```python
from build123d import *

# Parameters (mm, degrees)
SKETCH_1_R      = 1.05
SKETCH_1_W      = 7
SKETCH_1_H      = 5
SKETCH_1_W_2    = 5
SKETCH_1_H_2    = 11
SKETCH_1_W_3    = 21
SKETCH_1_H_3    = 2
SKETCH_1_R_2    = 8.5
EXTRUDE_1_DEPTH = 1.6


with BuildPart() as part:
    # 草图1 → 凸台-拉伸1 (new body)
    with BuildSketch(Plane(origin=(0, 0, 0), x_dir=(1, 0, 0), z_dir=(0, 1, 0))):
        Polygon((99, 0), (0, 0), (0, -143), (99, -143), (99, -93), (93, -93), (93, -80.5), (99, -80.5), align=None)
        with Locations(Location((21.8, -94.8, 0), (0, 0, 270))):
            Circle(SKETCH_1_R, mode=Mode.SUBTRACT)
        with Locations((73, -90.5)):
            Rectangle(SKETCH_1_W, SKETCH_1_H, mode=Mode.SUBTRACT)
        with Locations(Location((71.4, -77.5, 0), (0, 0, 270))):
            Circle(SKETCH_1_R, mode=Mode.SUBTRACT)
        with Locations(Location((94.8, -94.8, 0), (0, 0, 270))):
            Circle(SKETCH_1_R, mode=Mode.SUBTRACT)
        with Locations(Location((8.7, -65.7, 0), (0, 0, 270))):
            Circle(SKETCH_1_R, mode=Mode.SUBTRACT)
        with Locations((38, -39)):
            Rectangle(SKETCH_1_W_2, SKETCH_1_H_2, mode=Mode.SUBTRACT)
        with Locations(Location((21.8, -26.8, 0), (0, 0, 270))):
            Circle(SKETCH_1_R, mode=Mode.SUBTRACT)
        with Locations(Location((7, -7, 0), (0, 0, 270))):
            Circle(SKETCH_1_R, mode=Mode.SUBTRACT)
        with Locations(Location((20, -12, 0), (0, 0, 270))):
            Circle(SKETCH_1_R, mode=Mode.SUBTRACT)
        with Locations((24.5, -3)):
            Rectangle(SKETCH_1_W_3, SKETCH_1_H_3, mode=Mode.SUBTRACT)
        with Locations(Location((50, -36.3, 0), (0, 0, 270))):
            Circle(SKETCH_1_R_2, mode=Mode.SUBTRACT)
        with Locations(Location((96.3, -55.2, 0), (0, 0, 270))):
            Circle(SKETCH_1_R, mode=Mode.SUBTRACT)
        with Locations(Location((94.8, -26.8, 0), (0, 0, 270))):
            Circle(SKETCH_1_R, mode=Mode.SUBTRACT)
        with Locations(Location((81.9, -4.6, 0), (0, 0, 270))):
            Circle(SKETCH_1_R, mode=Mode.SUBTRACT)
        with Locations(Location((87, -7, 0), (0, 0, 270))):
            Circle(SKETCH_1_R, mode=Mode.SUBTRACT)
        with Locations(Location((66, -106, 0), (0, 0, 270))):
            Circle(SKETCH_1_R, mode=Mode.SUBTRACT)
        with Locations(Location((7, -136, 0), (0, 0, 270))):
            Circle(SKETCH_1_R, mode=Mode.SUBTRACT)
        with Locations(Location((33, -132, 0), (0, 0, 270))):
            Circle(SKETCH_1_R, mode=Mode.SUBTRACT)
        with Locations(Location((33, -106, 0), (0, 0, 270))):
            Circle(SKETCH_1_R, mode=Mode.SUBTRACT)
        with Locations(Location((66, -132, 0), (0, 0, 270))):
            Circle(SKETCH_1_R, mode=Mode.SUBTRACT)
        with Locations(Location((87, -136, 0), (0, 0, 270))):
            Circle(SKETCH_1_R, mode=Mode.SUBTRACT)
    extrude(amount=EXTRUDE_1_DEPTH)


solid = part.part
```
Verification items for the finished model (mm, model axes). Coordinates: 2 decimals unless noted, no trailing zeros. Loops run counter-clockwise (first coordinate to the right, second up) from the corner with the lowest first, then second, coordinate; pieces in that order, holes last. Notation, with made-up numbers: (56, -11) - (89, -11) arc R6 cw to (89, -4) - close; hole circle Ø9 at (10, 13.5). An arc over 180 degrees is marked (long way). Answer as a JSON object with one key per item and string values.
(1) Cross-section at B-B, the plane y = 1.1. Count the separate pieces of the cut face and the enclosed holes in it, then the cut area to 3 significant figures.
Response:
{"separate pieces": "1", "enclosed holes": "21", "area": "13,700 mm²"}
(2) Mould release check, pull along X, two halves, no side actions. Record for faces 1 (the flat face through (49, 0, 70)), 2 (the cylindrical face through (55.745, 0.789, 30.035)): pulls with the +X half, pulls with the -X half, needs draft (parallel to the pull), parting line crosses it, or undercut.
Response:
{"face 1": "needs draft", "face 2": "undercut"}
(3) Scan lines: line 1 along X through (y, z) = (0.75, 26.8); line 2 along X through (y, z) = (0.3, 7); line 3 along Z through (x, y) = (66, 0.65). Record each from-to range of solid material in increasing order.
Response:
{"line 1": "x = 0 to 20.75, 22.85 to 93.75, 95.85 to 99", "line 2": "x = 0 to 5.95, 8.05 to 85.95, 88.05 to 99", "line 3": "z = 0 to 104.95, 107.05 to 130.95, 133.05 to 143"}
(4) Go/stop test with flat-tipped pins: pin 1 Ø2.5 at (x, z) = (33, 132) entering from -Y; pin 2 Ø1.7 at (x, z) = (87, 7) entering from -Y. Record where each tip stops, or that it passes through.
Response:
{"pin 1": "stops at y = 0", "pin 2": "passes through"}
(5) Cross-section at A-A, the plane z = 42. Record the boundary of the cut face in (x, y).
Response:
{"outline": "(0, 0) - (35.5, 0) - (35.5, 1.6) - (0, 1.6) - close; (40.5, 0) - (43.69, 0) - (43.69, 1.6) - (40.5, 1.6) - close; (56.31, 0) - (99, 0) - (99, 1.6) - (56.31, 1.6) - close"}
